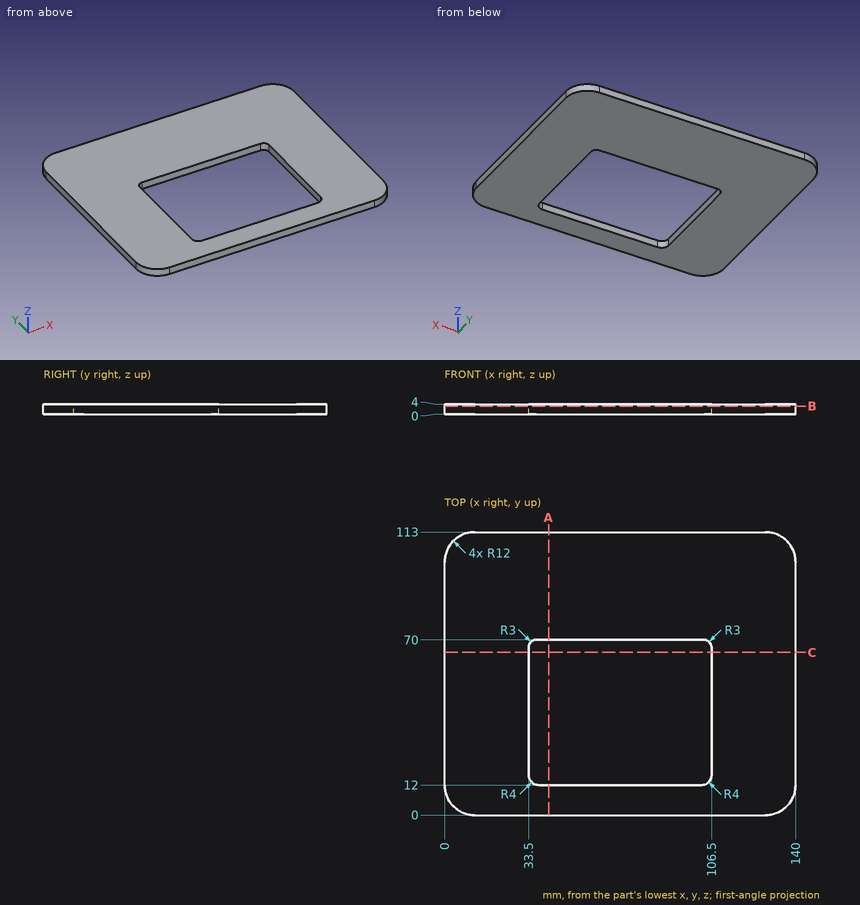
Could you check a few things on this drawing? It's one solid part, dimensions in mm from its lowest x, y, z. Give positions to 0.01 mm unless a question says otherwise; leave off trailing zeros. Order: outer loops, then holes, each group sorted by start corner. A loop starts at its lowest first (then second) coordinate and runs counter-clockwise, first axis right, second up. Notation, with made-up numbers: (-30.75, 24) - (-14.75, 24) arc R13 cw to (-14.75, 36) - close; hole circle Ø5 at (-4.75, 70.25). An arc over 180 degrees is marked (long way). One line per item, written item: value. Start each with the question number.
1. Imagine slicing it at B-B on z = 3.2. List the corners of the cut face in (x, y) for me.
2. Imagine slicing it at A-A on x = 41.5. List the corners of the cut face in (y, z) for me.
3. Imagine slicing it at C-C on y = 65. List the corners of the cut face in (x, z) for me, plus the area to 3 significant figures.
4. If I drill on probe 1 along Y at (x, z) = (38.5, 0.85); probe 2 along X at (y, z) = (50, 3); probe 3 along Y at (x, z) = (104, 0.9), over which ranges is the centre line in solid material (lowest first)?
Values:
1. outline: (0, 12) arc R12 ccw to (12, 0) - (128, 0) arc R12 ccw to (140, 12) - (140, 101) arc R12 ccw to (128, 113) - (12, 113) arc R12 ccw to (0, 101) - close; hole (33.5, 16) arc R4 ccw to (37.5, 12) - (102.5, 12) arc R4 ccw to (106.5, 16) - (106.5, 67) arc R3 ccw to (103.5, 70) - (36.5, 70) arc R3 ccw to (33.5, 67) - close
2. outline: (0, 0) - (12, 0) - (12, 4) - (0, 4) - close; (70, 0) - (113, 0) - (113, 4) - (70, 4) - close
3. outline: (0, 0) - (33.5, 0) - (33.5, 4) - (0, 4) - close; (106.5, 0) - (140, 0) - (140, 4) - (106.5, 4) - close
3. area: 268 mm²
4. probe 1: 0 to 12, 70 to 113
4. probe 2: 0 to 33.5, 106.5 to 140
4. probe 3: 0 to 12.29, 69.96 to 113
